from build123d import *

# Parameters (mm, degrees)
SKETCH1_R           = 11.8618
BOSS_EXTRUDE1_DEPTH = 1.4732
FILLET1_R           = 0.381


with BuildPart() as part:
    # Sketch1 → Boss-Extrude1 (new, symmetric)
    with BuildSketch(Plane(origin=(0, 0, 0), x_dir=(1, 0, 0), z_dir=(0, 1, 0))):
        with Locations(Location((0, 0, 0), (0, 0, 270))):
            Circle(SKETCH1_R)
        with BuildLine():
            Line((3.302250327, 5.207), (-3.302250327, 5.207))
            ThreePointArc((-3.302250327, 5.207), (-6.16585, 0), (-3.302250327, -5.207))
            Line((-3.302250327, -5.207), (3.302250327, -5.207))
            ThreePointArc((3.302250327, -5.207), (6.16585, 0), (3.302250327, 5.207))
        make_face(mode=Mode.SUBTRACT)
    extrude(amount=BOSS_EXTRUDE1_DEPTH, both=True)

    # Fillet1
    fillet1_edges = [part.edges().sort_by_distance(p)[0] for p in [
        (3.302250327, 0, -5.207),
        (-3.302250327, 0, -5.207),
        (-3.302250327, 0, 5.207),
        (3.302250327, 0, 5.207),
        (0, 1.4732, 5.207),
        (-6.16585, 1.4732, 0),
        (0, 1.4732, -5.207),
        (0, 1.4732, -11.8618),
        (6.16585, 1.4732, 0),
    ]]
    fillet(fillet1_edges, radius=FILLET1_R)


solid = part.part
Verification items for the finished model (mm, model axes). A direction names the side the tool comes from. Round coordinates to 2 decimals unless told otherwise and drop trailing zeros. Loops run counter-clockwise (first coordinate to the right, second up) from the corner with the lowest first, then second, coordinate; pieces in that order, holes last. Notation, with made-up numbers: (10.5, 8) - (66.5, 8) arc R23 ccw to (66.5, 47) - close; hole circle Ø11 at (-31, 14.25). An arc over 180 degrees is marked (long way). Answer in a Markdown table with one row per item. Add a question column.
Q1. Release check for a two-part mould opening along X. For faces 3 (the face through (0, 0, 5.207)), 4 (the face through (0.2, -1.473, -5.4)), 5 (the face through (3.563, -0.173, 11.314)) record: pulls with the +X half, pulls with the -X half, needs draft (parallel to the pull), parting line crosses it, or undercut.
Q2. Tool access check on faces 1 (the face through (-5, 1.473, 5)), 2 (the face through (0, 0, -5.207)). Record the directions out of +Z, -Z, +X, -X, +Y, -Y that give a thin tool (end or side, any length) a straight path to the whole face; none if there is none.
Q3. Section check B-B on z = 0. Enter the section's corners in (x, y).
Q4. Section check C-C on y = -0.3. Enter the section's corners in (x, z).
Q5. Material ranges on line 1 (Z direction, x = -3, y = 0.3); line 2 (Z direction, x = -3.5, y = -1.05); line 3 (X direction, y = 0.7, z = -4.5), recorded low to high.
Q6. Section check A-A on x = 0. Enter the section's corners in (y, z).
Q7. Gauge pin test, flat ends, axial feed: pin 1 (1 mm diameter, centred on x = 7, y = 0, fed in from +Z); pin 2 (1 mm diameter, centred on x = 3.5, z = -1.5, fed in from -Y); pin 3 (1 mm diameter, centred on x = -8, y = 0, fed in from +Z); pin 4 (1 mm diameter, centred on x = 6.5, y = 0, fed in from +Z). Record the tip position at first contact, or that the pin passes through.
Found:
| question | item | result |
|---|---|---|
| 1 | face 3 | undercut |
| 1 | face 4 | needs draft |
| 1 | face 5 | parting line crosses it |
| 2 | face 1 | +Z, -Z, +X, -X, +Y |
| 2 | face 2 | +Y, -Y |
| 3 | outline | (-11.86, -1.47) - (-6.17, -1.47) - (-6.17, 1.09) arc R0.38 ccw to (-6.55, 1.47) - (-11.48, 1.47) arc R0.38 ccw to (-11.86, 1.09) - close; (6.17, -1.47) - (11.86, -1.47) - (11.86, 1.09) arc R0.38 ccw to (11.48, 1.47) - (6.55, 1.47) arc R0.38 ccw to (6.17, 1.09) - close |
| 4 | outline | circle Ø23.72 at (0, 0); hole (-3.4, -5.14) arc R0.38 ccw to (-3.19, -5.21) - (3.19, -5.21) arc R0.38 ccw to (3.4, -5.14) arc R6.17 ccw to (3.4, 5.14) arc R0.38 ccw to (3.19, 5.21) - (-3.19, 5.21) arc R0.38 ccw to (-3.4, 5.14) arc R6.17 ccw to start |
| 5 | line 1 | z = -11.48 to -5.21, 5.21 to 11.48 |
| 5 | line 2 | z = -11.33 to -5.08, 5.08 to 11.33 |
| 5 | line 3 | x = -10.98 to -4.22, 4.22 to 10.98 |
| 6 | outline | (-1.47, -11.86) - (1.09, -11.86) arc R0.38 ccw to (1.47, -11.48) - (1.47, -5.59) arc R0.38 ccw to (1.09, -5.21) - (-1.47, -5.21) - close; (-1.47, 5.21) - (1.09, 5.21) arc R0.38 ccw to (1.47, 5.59) - (1.47, 11.48) arc R0.38 ccw to (1.09, 11.86) - (-1.47, 11.86) - close |
| 7 | pin 1 | stops at z = 9.92 |
| 7 | pin 2 | passes through |
| 7 | pin 3 | stops at z = 9.19 |
| 7 | pin 4 | stops at z = 10.23 |
